Can you work these out from the drawing? Everything is in mm from the part's minimum corner. A direction names the side the tool comes from. Round coordinates to 2 decimals unless told otherwise and drop trailing zeros. Order: outer loops, then holes, each group sorted by start corner. A loop starts at its lowest first (then second) coordinate and runs counter-clockwise, first axis right, second up. Notation, with made-up numbers: M 38,-24 L 77,-24 A10 ccw 77,-8 Z; hole C 4.25,60 d2. An arc over 180 degrees is marked long. Write each question's results on one line, items separated by ' | '. Start each with the question number.
1. Suppose I cut it at A-A on x = 90. Write out the boundary of the cut face in (y, z), and give its area (4 significant figures).
2. I'm going to push flat-ended pins straight in: pin 1 (8 mm diameter, centred on y = 19, z = 24.5, fed in from -X); pin 2 (6 mm diameter, centred on x = 8.5, y = 20, fed in from +Z); pin 3 (2 mm diameter, centred on y = 5.5, z = 28.5, fed in from +X); pin 4 (4.5 mm diameter, centred on x = 90, y = 15, fed in from +Z). Where does each tip first touch, or does it pass through?
3. Suppose I cut it at D-D on x = 50. Write out the boundary of the cut face in (y, z) (3 decimals).
4. Suppose I cut it at B-B on y = 15. Write out the boundary of the cut face in (x, z).
5. Suppose I cut it at C-C on z = 5. Write out the boundary of the cut face in (x, y).
6. Please list where these lines run through material, in increasing order: L1, parallel to X at y = 15, z = 7; L2, parallel to Y at x = 10, z = 11.5; L3, parallel to Y at x = 72, z = 10.
7. For the marked faces 1, 2, 3, 4 and 5, which set-ups out of +Z, -Z, +X, -X, +Y, -Y let a thin tool reach every point of the face, with its end or its side?
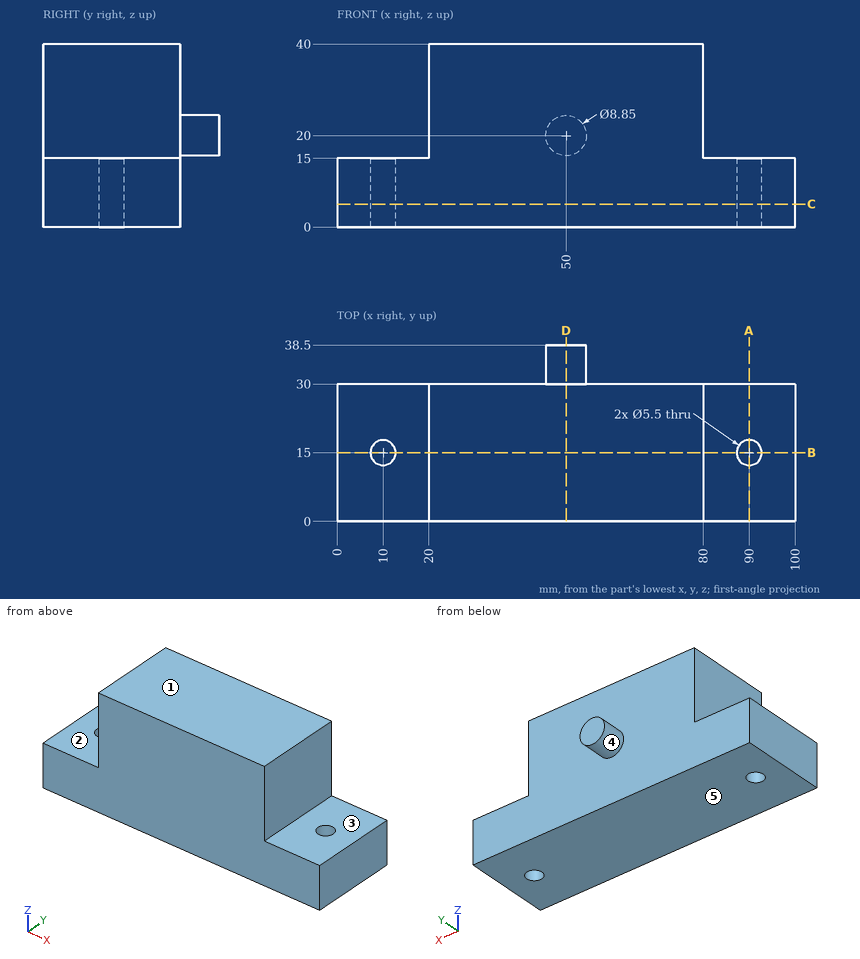
Filled sheet:
1) outline: M 0,0 L 12.25,0 L 12.25,15 L 0,15 Z; M 17.75,0 L 30,0 L 30,15 L 17.75,15 Z | area: 367.5 mm^2
2) pin 1: stops at x = 20 | pin 2: stops at z = 15 | pin 3: stops at x = 80 | pin 4: passes through
3) outline: M 0,0 L 30,0 L 30,15.575 L 38.5,15.575 L 38.5,24.425 L 30,24.425 L 30,40 L 0,40 Z
4) outline: M 0,0 L 7.25,0 L 7.25,15 L 0,15 Z; M 12.75,0 L 87.25,0 L 87.25,15 L 80,15 L 80,40 L 20,40 L 20,15 L 12.75,15 Z; M 92.75,0 L 100,0 L 100,15 L 92.75,15 Z
5) outline: M 0,0 L 100,0 L 100,30 L 0,30 Z; hole C 10,15 d5.5; hole C 90,15 d5.5
6) L1: x = 0 to 7.25, 12.75 to 87.25, 92.75 to 100 | L2: y = 0 to 12.25, 17.75 to 30 | L3: y = 0 to 30
7) face 1: +Z, +X, -X, +Y, -Y | face 2: +Z, -X, +Y, -Y | face 3: +Z, +X, +Y, -Y | face 4: +Y | face 5: -Z, +X, -X, +Y, -Y
